The listing builds one solid part. Answer for the finished solid, in the listing's coordinates (mm). Face numbers are marked on the shaded views. A direction names the side the tool comes from. Give positions to 0.01 mm unless a question says otherwise; leave off trailing zeros. Write each loop counter-clockwise with the first axis right and the second up, starting at its lowest first coordinate (ties: lowest second). Pieces come first, ordered by that corner, then holes. Notation, with made-up numbers: (61.25, 56) -> (68.25, 56) arc R35 ccw to (68.25, 90) -> close; hole circle Ø9 at (12, -20). An arc over 180 degrees is marked (long way). Write each question's results on one line, items separated by ' | '. Start each with the question number.
from build123d import *

# Parameters (mm, degrees)
SKETCH1_W           = 52
SKETCH1_H           = 95.5
BOSS_EXTRUDE1_DEPTH = 2
SKETCH2_R           = 1.6
CUT_EXTRUDE1_DEPTH  = 2
SKETCH3_W           = 52
SKETCH3_H           = 95.5
SKETCH3_W_2         = 48
SKETCH3_H_2         = 91.5
BOSS_EXTRUDE2_DEPTH = 35
SKETCH4_R           = 2.6
SKETCH4_R_2         = 1.6
BOSS_EXTRUDE3_DEPTH = 2


with BuildPart() as part:
    # Sketch1 → Boss-Extrude1 (new body)
    with BuildSketch(Plane(origin=(0, 0, 0), x_dir=(1, 0, 0), z_dir=(0, 1, 0))):
        Rectangle(SKETCH1_W, SKETCH1_H)
    extrude(amount=BOSS_EXTRUDE1_DEPTH)

    # Sketch2 → Cut-Extrude1 (cut)
    with BuildSketch(Plane(origin=(0, 2, 0), x_dir=(1, 0, 0), z_dir=(0, 1, 0))):
        with Locations((-16.85, 38.75)):
            Circle(SKETCH2_R)
        with Locations((16.85, 38.75)):
            Circle(SKETCH2_R)
        with Locations((-16.85, -38.75)):
            Circle(SKETCH2_R)
        with Locations((16.85, -38.75)):
            Circle(SKETCH2_R)
    extrude(amount=-CUT_EXTRUDE1_DEPTH, mode=Mode.SUBTRACT)

    # Sketch3 → Boss-Extrude2 (add)
    with BuildSketch(Plane(origin=(0, 2, 0), x_dir=(1, 0, 0), z_dir=(0, 1, 0))):
        Rectangle(SKETCH3_W, SKETCH3_H)
        Rectangle(SKETCH3_W_2, SKETCH3_H_2, mode=Mode.SUBTRACT)
    extrude(amount=BOSS_EXTRUDE2_DEPTH)

    # Sketch4 → Boss-Extrude3 (add)
    with BuildSketch(Plane(origin=(0, 2, 0), x_dir=(1, 0, 0), z_dir=(0, 1, 0))):
        with Locations((-16.85, 38.75)):
            Circle(SKETCH4_R)
        with Locations((-16.85, 38.75)):
            Circle(SKETCH4_R_2, mode=Mode.SUBTRACT)
        with Locations((16.85, 38.75)):
            Circle(SKETCH4_R)
        with Locations((16.85, 38.75)):
            Circle(SKETCH4_R_2, mode=Mode.SUBTRACT)
        with Locations((16.85, -38.75)):
            Circle(SKETCH4_R)
        with Locations((16.85, -38.75)):
            Circle(SKETCH4_R_2, mode=Mode.SUBTRACT)
        with Locations((-16.85, -38.75)):
            Circle(SKETCH4_R)
        with Locations((-16.85, -38.75)):
            Circle(SKETCH4_R_2, mode=Mode.SUBTRACT)
    extrude(amount=BOSS_EXTRUDE3_DEPTH)


solid = part.part
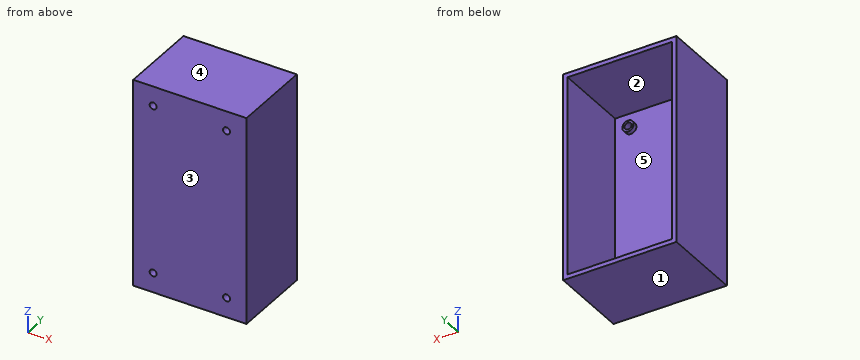
1. Section C-C (x = 3.5) is taken. Write down the section's boundary in (y, z).
2. Consider probe 1 along X at (y, z) = (2.4, 38.75); probe 2 along Z at (x, y) = (16.85, 1.4); probe 3 along X at (y, z) = (4.5, -28). Determine where each line is inside the solid, lowest interval first. Write a range as [from, to].
3. Each of these flat-tipped pins is pushed along its axis until it touches: pin 1 Ø4 at (x, z) = (-16.5, -39) entering from +Y; pin 2 Ø6 at (x, z) = (12.5, 12) entering from +Y; pin 3 Ø3 at (x, z) = (-16.85, 38.75) entering from +Y. Where does it stop, or does it pass through?
4. A tool of negligible diameter and unlimited length cuts with its end or side. For the marked faces 4 and 5, from which of +Z, -Z, +X, -X, +Y, -Y can it reach the whole face along a straight path? Write none if from no direction.
5. Section D-D (y = 25.5) is taken. Write down the section's boundary in (x, z).
6. The mould has two halves that part along Z. Classify the marked faces 1, 2 and 3: pulls with the +Z half, pulls with the -Z half, needs draft (parallel to the pull), parting line crosses it, or undercut.
7. Section A-A (z = 38.75) is taken. Write down the section's boundary in (x, y).
8. Section B-B (x = -16.85) is taken. Write down the section's boundary in (y, z).
Results:
1) outline: (0, -47.75) -> (37, -47.75) -> (37, -45.75) -> (2, -45.75) -> (2, 45.75) -> (37, 45.75) -> (37, 47.75) -> (0, 47.75) -> close
2) probe 1: x = [-26, -24], [-19.45, -18.45], [-15.25, -14.25], [14.25, 15.25], [18.45, 19.45], [24, 26] | probe 2: z = [-47.75, -40.35], [-37.15, 37.15], [40.35, 47.75] | probe 3: x = [-26, -24], [24, 26]
3) pin 1: stops at y = 4 | pin 2: stops at y = 2 | pin 3: passes through
4) face 4: +Z, +X, -X, +Y, -Y | face 5: +Y
5) outline: (-26, -47.75) -> (26, -47.75) -> (26, 47.75) -> (-26, 47.75) -> close; hole (-24, -45.75) -> (24, -45.75) -> (24, 45.75) -> (-24, 45.75) -> close
6) face 1: pulls with the -Z half | face 2: undercut | face 3: needs draft
7) outline: (-26, 0) -> (-18.45, 0) -> (-18.45, 4) -> (-19.45, 4) -> (-19.45, 2) -> (-24, 2) -> (-24, 37) -> (-26, 37) -> close; (-15.25, 0) -> (15.25, 0) -> (15.25, 4) -> (14.25, 4) -> (14.25, 2) -> (-14.25, 2) -> (-14.25, 4) -> (-15.25, 4) -> close; (18.45, 0) -> (26, 0) -> (26, 37) -> (24, 37) -> (24, 2) -> (19.45, 2) -> (19.45, 4) -> (18.45, 4) -> close
8) outline: (0, -47.75) -> (37, -47.75) -> (37, -45.75) -> (2, -45.75) -> (2, -41.35) -> (4, -41.35) -> (4, -40.35) -> (0, -40.35) -> close; (0, -37.15) -> (4, -37.15) -> (4, -36.15) -> (2, -36.15) -> (2, 36.15) -> (4, 36.15) -> (4, 37.15) -> (0, 37.15) -> close; (0, 40.35) -> (4, 40.35) -> (4, 41.35) -> (2, 41.35) -> (2, 45.75) -> (37, 45.75) -> (37, 47.75) -> (0, 47.75) -> close
